CAD build for the part. Positions are in the model's coordinates, mm. Face numbers are marked on the shaded views. Coordinates: 2 decimals unless noted, no trailing zeros. Write each loop counter-clockwise with the first axis right and the second up, starting at its lowest first coordinate (ties: lowest second). Pieces come first, ordered by that corner, then holes. Notation, with made-up numbers: (78, 37.25) - (137, 37.25) arc R16 cw to (137, 60.25) - close; hole circle Ø1 at (-38.5, -28). An arc over 180 degrees is marked (long way). Answer in a Markdown table with one row per item. Add a question column.
Q1. Pin check, flat tips, straight feed: pin 1 (1 mm diameter, centred on x = 34.5, y = -1, fed in from -Z); pin 2 (4 mm diameter, centred on x = -11.5, z = 21.5, fed in from +Y); pin 3 (12 mm diameter, centred on x = 28, y = -20, fed in from -Z). Stop position of each tip, or through.
Q2. Band-saw the part on A-A (y = 0). List the corners of the cut face in (x, z), and give its area (3 significant figures).
Q3. Drill centre lines: line 1 along Y through (x, z) = (23, 0); line 2 along Z through (x, y) = (3.5, 1); line 3 along X through (y, z) = (-16.5, 26). Where is each one in solid material? Low to high. Write a range as from..to.
Q4. Band-saw the part on C-C (x = 41). List the corners of the cut face in (y, z).
Q5. Band-saw the part on D-D (x = 2). List the corners of the cut face in (y, z), and give its area (3 significant figures).
Q6. Two-plate mould, pull along Z, no slides. Class the marked faces 1, 2, 3 and 4: +Z half, -Z half, draft (parallel to the pull), parting line (faces both ways), or undercut.
```python
from build123d import *

# Parameters (mm, degrees)
SKETCH1_R           = 42.5
BOSS_EXTRUDE1_DEPTH = 50
SKETCH6_R           = 40
CUT_EXTRUDE6_DEPTH  = 35
SKETCH9_R           = 42.5
CUT_EXTRUDE12_DEPTH = 20


with BuildPart() as part:
    # Sketch1 → Boss-Extrude1 (new body, symmetric)
    with BuildSketch(Plane(origin=(0, 0, 0), x_dir=(0, 0, -1), z_dir=(1, 0, 0))):
        Circle(SKETCH1_R)
    extrude(amount=BOSS_EXTRUDE1_DEPTH, both=True)

    # Sketch6 → Cut-Extrude6 (cut)
    with BuildSketch(Plane(origin=(50, 0, 0), x_dir=(0, 0, -1), z_dir=(1, 0, 0))):
        Circle(SKETCH6_R)
    extrude(amount=-CUT_EXTRUDE6_DEPTH, mode=Mode.SUBTRACT)

    # Sketch9 → Cut-Extrude12 (cut)
    with BuildSketch(Plane.ZY.offset(50)):
        Circle(SKETCH9_R)
    extrude(amount=-CUT_EXTRUDE12_DEPTH, mode=Mode.SUBTRACT)


solid = part.part
```
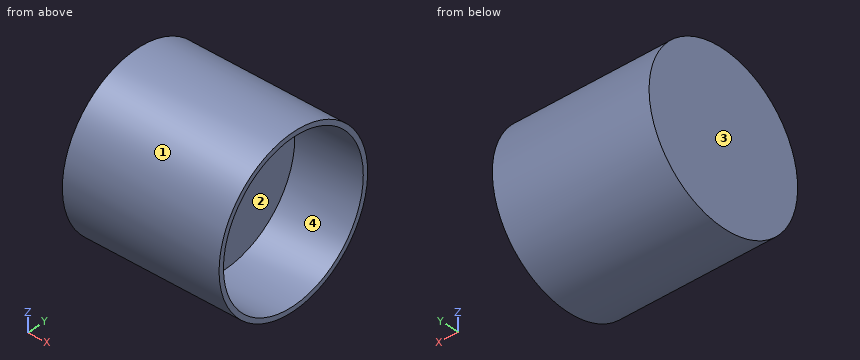
Checked values:
| question | item | result |
|---|---|---|
| 1 | pin 1 | stops at z = -42.5 |
| 1 | pin 2 | stops at y = 37.76 |
| 1 | pin 3 | stops at z = -40.13 |
| 2 | outline | (-30, -42.5) - (50, -42.5) - (50, -40) - (15, -40) - (15, 40) - (50, 40) - (50, 42.5) - (-30, 42.5) - close |
| 2 | area | 4,000 mm² |
| 3 | line 1 | y = -42.5..-40, 40..42.5 |
| 3 | line 2 | z = -42.49..42.49 |
| 3 | line 3 | x = -30..15 |
| 4 | outline | circle Ø85 at (0, 0); hole circle Ø80 at (0, 0) |
| 5 | outline | circle Ø85 at (0, 0) |
| 5 | area | 5,670 mm² |
| 6 | face 1 | parting line |
| 6 | face 2 | undercut |
| 6 | face 3 | draft |
| 6 | face 4 | undercut |
